Part model, mm, in its own coordinate system. Coordinates: 2 decimals unless noted, no trailing zeros. Write each loop counter-clockwise with the first axis right and the second up, starting at its lowest first coordinate (ties: lowest second). Pieces come first, ordered by that corner, then holes. Notation, with made-up numbers: (18, 88.5) - (68, 88.5) arc R19 ccw to (68, 123.5) - close; hole circle Ø4 at (70.25, 8.25). An arc over 180 degrees is marked (long way). Use one line per item in the form item = value. Start each with the question number.
from build123d import *

# Parameters (mm, degrees)
STOP_PLATE_BLANK_SKETCH_W    = 2
STOP_PLATE_BLANK_SKETCH_H    = 3.6
STOP_PLATE_BLANK_DEPTH       = 20
M2_STOP_CLEARANCE_1_SKETCH_R = 1.2
M2_STOP_CLEARANCE_1_DEPTH    = 2.2
M2_STOP_CLEARANCE_2_SKETCH_R = 1.2
M2_STOP_CLEARANCE_2_DEPTH    = 2.2


with BuildPart() as part:
    # Stop plate blank sketch → Stop plate blank (new body)
    with BuildSketch(Plane.XY.offset(-38)):
        with Locations((24.708348754, -61.4)):
            Rectangle(STOP_PLATE_BLANK_SKETCH_W, STOP_PLATE_BLANK_SKETCH_H)
    extrude(amount=STOP_PLATE_BLANK_DEPTH)

    # M2 stop clearance 1 sketch → M2 stop clearance 1 (cut)
    with BuildSketch(Plane(origin=(23.608348754, 0, 0), x_dir=(0, 0, -1), z_dir=(1, 0, 0))):
        with Locations(Location((34, -61.4, 0), (0, 0, 180))):
            Circle(M2_STOP_CLEARANCE_1_SKETCH_R)
    extrude(amount=M2_STOP_CLEARANCE_1_DEPTH, mode=Mode.SUBTRACT)

    # M2 stop clearance 2 sketch → M2 stop clearance 2 (cut)
    with BuildSketch(Plane(origin=(23.608348754, 0, 0), x_dir=(0, 0, -1), z_dir=(1, 0, 0))):
        with Locations(Location((28, -61.4, 0), (0, 0, 180))):
            Circle(M2_STOP_CLEARANCE_2_SKETCH_R)
    extrude(amount=M2_STOP_CLEARANCE_2_DEPTH, mode=Mode.SUBTRACT)


solid = part.part
Q1. Slice it at A-A (z = -28). List the corners of the cut face in (x, y), plus the area to 3 significant figures.
Q2. Drill centre lines: probe 1 along Z at (x, y) = (24.7, -61.3); probe 2 along Y at (x, z) = (24.65, -34); probe 3 along Z at (x, y) = (25.65, -62.2). Where is each one in solid material? Low to high.
Q3. Slice it at C-C (x = 25.2). List the corners of the cut face in (y, z).
Q4. Slice it at B-B (y = -61.9). List the corners of the cut face in (x, z).
Q5. Pin check, flat tip, straight feed: P1, Ø1.9, axis at y = -61.4, z = -34, coming from the +X side. Stop position of the tip, or through.
Q6. Mould opens along Z. For faces 1 (the flat face through (25, -61, -38)), 2 (the cylindrical face through (24.694, -60.335, -33.446)), 3 (the flat face through (25, -63.2, -28)), 4 (the flat face through (25, -61, -18)) say: released by +Z, released by -Z, zero draft, split by the parting line, or undercut.
Solution:
q1.outline = (23.71, -63.2) - (25.71, -63.2) - (25.71, -62.6) - (23.71, -62.6) - close; (23.71, -60.2) - (25.71, -60.2) - (25.71, -59.6) - (23.71, -59.6) - close
q1.area = 2.40 mm2
q2.probe_1 = -38 to -35.2, -32.8 to -29.2, -26.8 to -18
q2.probe_2 = -63.2 to -62.6, -60.2 to -59.6
q2.probe_3 = -38 to -34.89, -33.11 to -28.89, -27.11 to -18
q3.outline = (-63.2, -38) - (-59.6, -38) - (-59.6, -18) - (-63.2, -18) - close; hole circle Ø2.4 at (-61.4, -34); hole circle Ø2.4 at (-61.4, -28)
q4.outline = (23.71, -38) - (25.71, -38) - (25.71, -35.09) - (23.71, -35.09) - close; (23.71, -32.91) - (25.71, -32.91) - (25.71, -29.09) - (23.71, -29.09) - close; (23.71, -26.91) - (25.71, -26.91) - (25.71, -18) - (23.71, -18) - close
q5.P1 = through
q6.face_1 = released by -Z
q6.face_2 = undercut
q6.face_3 = zero draft
q6.face_4 = released by +Z
